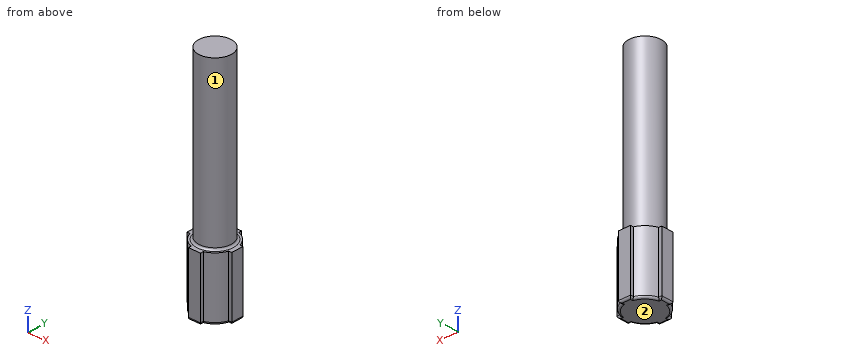
```python
from build123d import *

# Parameters (mm, degrees)
SKETCH1_R           = 9.95
SKETCH1_W           = 6
SKETCH1_H           = 21.99
SKETCH1_W_2         = 21.99
SKETCH1_H_2         = 6
BOSS_EXTRUDE1_DEPTH = 15
SKETCH2_R           = 8
BOSS_EXTRUDE2_DEPTH = 80
FILLET1_R           = 1


with BuildPart() as part:
    # Sketch1 → Boss-Extrude1 (new, symmetric)
    with BuildSketch(Plane.XY):
        Circle(SKETCH1_R)
        Rectangle(SKETCH1_W, SKETCH1_H)
        Rectangle(SKETCH1_W_2, SKETCH1_H_2)
    extrude(amount=BOSS_EXTRUDE1_DEPTH, both=True)

    # Sketch2 → Boss-Extrude2 (add)
    with BuildSketch(Plane.XY.offset(15)):
        Circle(SKETCH2_R)
    extrude(amount=BOSS_EXTRUDE2_DEPTH)

    # Fillet1
    fillet1_edges = [part.edges().sort_by_distance(p)[0] for p in [
        (10.240982371, 3, -15),
        (10.995, 0, -15),
        (10.240982371, -3, -15),
        (-3, 10.240982371, -15),
        (0, 10.995, -15),
        (3, 10.240982371, -15),
        (3, -10.240982371, -15),
        (0, -10.995, -15),
        (-3, -10.240982371, -15),
        (7.035712473, -7.035712473, -15),
        (7.035712473, 7.035712473, -15),
        (-7.035712473, 7.035712473, -15),
        (-7.035712473, -7.035712473, -15),
        (-8, 0, 15),
        (-10.240982371, -3, -15),
        (-10.995, 0, -15),
        (-10.240982371, 3, -15),
    ]]
    fillet(fillet1_edges, radius=FILLET1_R)


solid = part.part
```
Source: CAD feature listing. Evaluate the final solid. Frame: model axes, mm. Face numbers are marked on the shaded views. A direction names the side the tool comes from. Round coordinates to 2 decimals unless told otherwise and drop trailing zeros. Order: outer loops, then holes, each group sorted by start corner. A loop starts at its lowest first (then second) coordinate and runs counter-clockwise, first axis right, second up. Notation, with made-up numbers: (8.5, 6) -> (29.5, 6) arc R21 cw to (29.5, 17) -> close; hole circle Ø6 at (84, 66). An arc over 180 degrees is marked (long way). One line per item, written item: value. Start each with the question number.
Q1. Section query A-A (x = 0). Return the cut outline in (y, z) (3 decimals).
Q2. Pin query (flat end, axial travel): pin 1 (1.5 mm diameter, centred on x = -8.5, y = 8.5, fed in from +Z); pin 2 (0.8 mm diameter, centred on y = 10, z = 4, fed in from +X); pin 3 (0.5 mm diameter, centred on x = -10.5, z = 6, fed in from -Y); pin 4 (1.7 mm diameter, centred on x = -10.5, z = 3.5, fed in from +Y). Return the tip coordinate at first contact, or that it passes through.
Q3. Section query C-C (z = 21). Return the cut outline in (x, y), plus the area to 3 significant figures.
Q4. Material intervals for probe 1 along Y at (x, z) = (-0.5, 74.5); probe 2 along X at (y, z) = (9.5, 3.5), sorted ascending.
Q5. Access query for the marked faces 1 and 2. Directions: +Z, -Z, +X, -X, +Y, -Y. A direction counts if a zero-diameter tool reaches every point of the face in a straight line with its end or side. Return the directions, or none.
Findings below:
1. outline: (-10.995, -14) arc R1 ccw to (-9.995, -15) -> (9.995, -15) arc R1 ccw to (10.995, -14) -> (10.995, 15) -> (9, 15) arc R1 cw to (8, 16) -> (8, 95) -> (-8, 95) -> (-8, 16) arc R1 cw to (-9, 15) -> (-10.995, 15) -> close
2. pin 1: through
2. pin 2: x = 3
2. pin 3: y = -3
2. pin 4: y = 3
3. outline: circle Ø16 at (0, 0)
3. area: 201 mm²
4. probe 1: -7.98 to 7.98
4. probe 2: -3 to 3
5. face 1: +Z
5. face 2: -Z, +X, -X, +Y, -Y
